Geometry: final body of the model. Coordinates: model frame, mm. Give positions to 0.01 mm unless a question says otherwise; leave off trailing zeros. Write each loop counter-clockwise with the first axis right and the second up, starting at its lowest first coordinate (ties: lowest second). Pieces come first, ordered by that corner, then holes. Notation, with made-up numbers: M -15.75,-36.75 L 39.25,-36.75 A17 cw 39.25,-28.75 Z; hole C 4.5,-30 d11. An arc over 180 degrees is marked long. Use a Markdown table: item, result. Add a question column.
(1) Cut plane B-B (y = 86). Output: boundary loops of the cut face in (x, z) (3 decimals), plus the area to 3 significant figures.
(2) Cut plane A-A (z = 0.55). Output: boundary loops of the cut face in (x, y) (3 decimals), plus the area to 3 significant figures.
(3) Pin query (flat end, axial travel): pin 1 Ø1.5 at (x, z) = (47, 0.5) entering from -Y; pin 2 Ø1.6 at (y, z) = (116, 2) entering from -X; pin 3 Ø8 at (x, y) = (46, 66.5) entering from -Z; pin 4 Ø1.6 at (x, z) = (51, 1.5) entering from +Y. Return the tip coordinate at first contact, or that it passes through.
(4) Material intervals for L1, parallel to X at y = 72, z = 1.5; L2, parallel to Y at x = 11, z = 1.3, sorted ascending.
(5) Cut plane C-C (x = 14). Output: boundary loops of the cut face in (y, z) (3 decimals), plus the area to 3 significant figures.
Autodesk Inventor part; units mm, degrees
ref_plane "YZ Plane" through (0, 0, 0) normal (1, 0, 0) x (0, 1, 0)
ref_plane "XZ Plane" through (0, 0, 0) normal (0, 1, 0) x (-1, 0, 0)
ref_plane "XY Plane" through (0, 0, 0) normal (0, 0, 1) x (1, 0, 0)
sketch "Sketch1" plane through (0, 0, 0) normal (0, 0, 1) x (1, 0, 0)
  line L0 (0, 0) -> (52.9336, 0)
  line L1 (52.9336, 0) -> (52.9336, 114.3)
  line L2 (52.9336, 114.3) -> (0, 114.3)
  line L3 (0, 114.3) -> (0, 0)
  dimension "d0" = 114.3
  dimension "d1" = 52.9336
extrude "Extrusion1" add sketch "Sketch1" along normal blind 3.175
sketch "Sketch2" plane through (0, 0, 3.175) normal (0, 0, 1) x (1, 0, 0)
  line L0 (0, 114.3) -> (0, 0)
  line L1 (52.9336, 0) -> (52.9336, 114.3)
  line L2 (0, 60.96) -> (-3.175, 60.96)
  line L3 (-3.175, 60.96) -> (-3.175, 53.34)
  line L4 (-3.175, 53.34) -> (0, 53.34)
  line L5 (0, 53.34) -> (0, 60.96)
  line L6 (52.9336, 60.96) -> (49.7586, 60.96)
  line L7 (49.7586, 60.96) -> (49.7586, 53.34)
  line L8 (49.7586, 53.34) -> (52.9336, 53.34)
  line L9 (52.9336, 53.34) -> (52.9336, 60.96)
  line L10 (52.9336, 114.3) -> (0, 114.3)
  line L11 (0, 0) -> (52.9336, 0)
  line L12 (22.6568, 114.3) -> (22.6568, 117.475)
  line L13 (22.6568, 117.475) -> (30.2768, 117.475)
  line L14 (30.2768, 117.475) -> (30.2768, 114.3)
  line L15 (30.2768, 114.3) -> (22.6568, 114.3)
  line L16 (30.2768, 0) -> (30.2768, -3.175)
  line L17 (30.2768, -3.175) -> (22.6568, -3.175)
  line L18 (22.6568, -3.175) -> (22.6568, 0)
  line L19 (22.6568, 0) -> (30.2768, 0)
  point P0 (0, 57.15)
  point P1 (52.9336, 57.15)
  point P2 (26.4668, 114.3)
  point P3 (26.4668, 0)
  dimension "d4" = 3.81
  dimension "d5" = 7.62
  dimension "d6" = 3.175
  dimension "d7" = 3.81
  dimension "d8" = 7.62
  dimension "d9" = 3.175
  dimension "d10" = 3.81
  dimension "d11" = 3.81
  dimension "d12" = 3.175
  dimension "d13" = 7.62
  dimension "d14" = 3.81
  dimension "d15" = 3.175
extrude "Extrusion2" add sketch "Sketch2" against normal blind 3.175 contours L0 L4 L3 L2 | L12 L13 L14 L10 | L11 L16 L17 L18 | L1 L8 L7 L6
extrude "Extrusion3" cut sketch "Sketch2" against normal blind 3.175 contours L1 L8 L7 L6
properties part number "Birdhouse Wall"
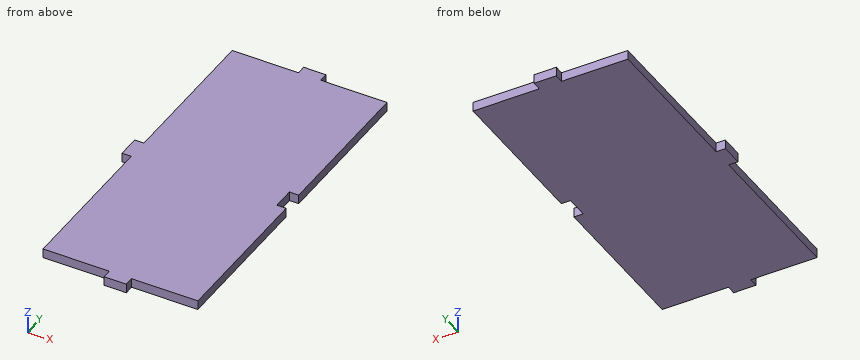
Answer list:
| question | item | result |
|---|---|---|
| 1 | outline | M 0,0 L 52.934,0 L 52.934,3.175 L 0,3.175 Z |
| 1 | area | 168 mm² |
| 2 | outline | M -3.175,53.34 L 0,53.34 L 0,0 L 22.657,0 L 22.657,-3.175 L 30.277,-3.175 L 30.277,0 L 52.934,0 L 52.934,53.34 L 49.759,53.34 L 49.759,60.96 L 52.934,60.96 L 52.934,114.3 L 30.277,114.3 L 30.277,117.475 L 22.657,117.475 L 22.657,114.3 L 0,114.3 L 0,60.96 L -3.175,60.96 Z |
| 2 | area | 6,100 mm² |
| 3 | pin 1 | y = 0 |
| 3 | pin 2 | x = 22.66 |
| 3 | pin 3 | z = 0 |
| 3 | pin 4 | y = 114.3 |
| 4 | L1 | 0 to 52.93 |
| 4 | L2 | 0 to 114.3 |
| 5 | outline | M 0,0 L 114.3,0 L 114.3,3.175 L 0,3.175 Z |
| 5 | area | 363 mm² |
